Here's how the part is built. I have some questions about the finished solid (model axes, mm). A direction names the side the tool comes from. Round coordinates to 2 decimals unless told otherwise and drop trailing zeros. Order: outer loops, then holes, each group sorted by start corner. A loop starts at its lowest first (then second) coordinate and runs counter-clockwise, first axis right, second up. Notation, with made-up numbers: (83, 32) - (127, 32) arc R25 ccw to (127, 55) - close; hole circle Ø5 at (74.5, 23). An arc over 180 degrees is marked (long way). Answer as a JSON object with one key per item and string values.
```python
from build123d import *

# Parameters (mm, degrees)
SKETCH1_W           = 22.7
SKETCH1_H           = 44.5
BOSS_EXTRUDE1_DEPTH = 2
SKETCH2_W           = 22.7
SKETCH2_H           = 44.5
SKETCH2_W_2         = 18.7
SKETCH2_H_2         = 40.5
BOSS_EXTRUDE2_DEPTH = 3
SKETCH3_W           = 5
SKETCH3_H           = 3
SKETCH3_W_2         = 4.1
SKETCH3_R           = 1.4
BOSS_EXTRUDE3_DEPTH = 5
SKETCH4_W           = 2
SKETCH4_H           = 5
CUT_EXTRUDE1_DEPTH  = 3
CUT_EXTRUDE2_DEPTH  = 3
FILLET2_R           = 1
SKETCH12_W          = 13.7
SKETCH12_H          = 18.15
SKETCH12_H_2        = 4.85
BOSS_EXTRUDE8_DEPTH = 3
CUT_EXTRUDE3_DEPTH  = 3


with BuildPart() as part:
    # Sketch1 → Boss-Extrude1 (new body)
    with BuildSketch(Plane.XY):
        Rectangle(SKETCH1_W, SKETCH1_H)
    extrude(amount=BOSS_EXTRUDE1_DEPTH)

    # Sketch2 → Boss-Extrude2 (add)
    with BuildSketch(Plane.XY.offset(2)):
        Rectangle(SKETCH2_W, SKETCH2_H)
        Rectangle(SKETCH2_W_2, SKETCH2_H_2, mode=Mode.SUBTRACT)
    extrude(amount=BOSS_EXTRUDE2_DEPTH)

    # Sketch3 → Boss-Extrude3 (add)
    with BuildSketch(Plane.XY.offset(2)):
        with Locations((6.85, -14.25)):
            Rectangle(SKETCH3_W, SKETCH3_H)
        with Locations((-7.3, -14.25)):
            Rectangle(SKETCH3_W_2, SKETCH3_H)
        with Locations((0, -2.9)):
            Circle(SKETCH3_R)
    extrude(amount=BOSS_EXTRUDE3_DEPTH)

    # Sketch4 → Cut-Extrude1 (cut, through all)
    with BuildSketch(Plane(origin=(-9.35, 0, 0), x_dir=(0, 0, -1), z_dir=(1, 0, 0))):
        with Locations((-3, -2.5)):
            Rectangle(SKETCH4_W, SKETCH4_H)
    extrude(amount=-CUT_EXTRUDE1_DEPTH, mode=Mode.SUBTRACT)

    # Sketch8 → Cut-Extrude2 (cut, through all)
    with BuildSketch(Plane.ZY.offset(-9.35)):
        Polygon((2, 0), (2, -2.5), (2, -5), (4, -5), (4, -2.5), (4, 0), align=None)
    extrude(amount=-CUT_EXTRUDE2_DEPTH, mode=Mode.SUBTRACT)

    # Fillet2
    fillet2_edges = [part.edges().sort_by_distance(p)[0] for p in [
        (0, -22.25, 0),
        (-11.35, 0, 0),
        (0, 22.25, 0),
        (11.35, 0, 0),
        (11.35, -22.25, 2.5),
        (-11.35, -22.25, 2.5),
        (-11.35, 22.25, 2.5),
        (11.35, 22.25, 2.5),
    ]]
    fillet(fillet2_edges, radius=FILLET2_R)

    # Sketch12 → Boss-Extrude8 (add)
    with BuildSketch(Plane.XY.offset(2)):
        with Locations((0, 8.675)):
            Rectangle(SKETCH12_W, SKETCH12_H)
        with Locations((0, -7.825)):
            Rectangle(SKETCH12_W, SKETCH12_H_2)
    extrude(amount=BOSS_EXTRUDE8_DEPTH)

    # Sketch13 → Cut-Extrude3 (cut, through all)
    with BuildSketch(Plane(origin=(0, -20.25, 0), x_dir=(1, 0, 0), z_dir=(0, 1, 0))):
        with BuildLine():
            Line((-2.5, -5), (2.5, -5))
            ThreePointArc((2.5, -5), (0, -2.5), (-2.5, -5))
        make_face()
    extrude(amount=-CUT_EXTRUDE3_DEPTH, mode=Mode.SUBTRACT)


solid = part.part
```
1. Imagine slicing it at A-A (z = 6.5). List the corners of the cut face in (x, y) for me, plus the area to 3 significant figures.
Responses:
{"outline": "(-9.35, -15.75) - (-5.25, -15.75) - (-5.25, -12.75) - (-9.35, -12.75) - close; circle Ø2.8 at (0, -2.9); (4.35, -15.75) - (9.35, -15.75) - (9.35, -12.75) - (4.35, -12.75) - close", "area": "33.5 mm2"}
2. Thinking about a two-plate mould opening in Y: for faces 6 (the face through (-7, -14, 7)), 7 (the face through (0, 22.25, 3)), 8 (the face through (-9.35, -18, 3)), which applies, pulls with the +Y half, pulls with the -Y half, needs draft (parallel to the pull), parting line crosses it, or undercut?
Responses:
{"face 6": "needs draft", "face 7": "pulls with the +Y half", "face 8": "undercut"}
3. For P1, Ø4, axis at x = -2.5, y = -8, coming from the +Z side; P2, Ø1.5, axis at x = 6, z = 6.5, coming from the +Y side, each with a flat end and sliding along its axis, tell me the tip position at first contact or that it passes through.
Responses:
{"P1": "z = 5", "P2": "y = -12.75"}
4. Imagine slicing it at C-C (x = 0). List the corners of the cut face in (y, z) for me, plus the area to 3 significant figures.
Responses:
{"outline": "(-22.25, 1) arc R1 ccw to (-21.25, 0) - (21.25, 0) arc R1 ccw to (22.25, 1) - (22.25, 5) - (20.25, 5) - (20.25, 2) - (17.75, 2) - (17.75, 5) - (-0.4, 5) - (-0.4, 2) - (-1.5, 2) - (-1.5, 7) - (-4.3, 7) - (-4.3, 2) - (-5.4, 2) - (-5.4, 5) - (-10.25, 5) - (-10.25, 2) - (-20.25, 2) - (-20.25, 2.5) - (-22.25, 2.5) - close", "area": "179 mm2"}
5. Imagine slicing it at B-B (y = -2.9). List the corners of the cut face in (x, z) for me.
Responses:
{"outline": "(-11.35, 1) arc R1 ccw to (-10.35, 0) - (10.35, 0) arc R1 ccw to (11.35, 1) - (11.35, 2) - (1.4, 2) - (1.4, 7) - (-1.4, 7) - (-1.4, 2) - (-11.35, 2) - close; (-11.35, 4) - (-9.35, 4) - (-9.35, 5) - (-11.35, 5) - close; (9.35, 4) - (11.35, 4) - (11.35, 5) - (9.35, 5) - close"}
6. Imagine slicing it at D-D (y = 6.5). List the corners of the cut face in (x, z) for me, plus the area to 3 significant figures.
Responses:
{"outline": "(-11.35, 1) arc R1 ccw to (-10.35, 0) - (10.35, 0) arc R1 ccw to (11.35, 1) - (11.35, 5) - (9.35, 5) - (9.35, 2) - (6.85, 2) - (6.85, 5) - (-6.85, 5) - (-6.85, 2) - (-9.35, 2) - (-9.35, 5) - (-11.35, 5) - close", "area": "98.1 mm2"}
7. If I drill on L1, parallel to Y at x = -3.25, z = 2.25; L2, parallel to Y at x = -8.5, z = 2.25; L3, parallel to X at y = 6.5, z = 2.25, over which ranges is the centre line in solid material (lowest first)? Write a range as [from, to].
Responses:
{"L1": "[-22.25, -20.25], [-10.25, -5.4], [-0.4, 17.75], [20.25, 22.25]", "L2": "[-22.25, -20.25], [-15.75, -12.75], [20.25, 22.25]", "L3": "[-11.35, -9.35], [-6.85, 6.85], [9.35, 11.35]"}
8. For faces 1 (the face through (-10, -5, 3)), 2 (the face through (0.1, -21.2, 2.5)), 3 (the face through (10, -3, 4)), 4 (the face through (6.85, 9, 3)), 5 (the face through (-10, 0, 3)), which set-ups out of +Z, -Z, +X, -X, +Y, -Y let a thin tool reach every point of the face, with its end or its side?
Responses:
{"face 1": "+X, -X", "face 2": "+Z, -Y", "face 3": "+X", "face 4": "+Z", "face 5": "-X"}
